Model file for the job. Use its own axes, mm. Face numbers are marked on the shaded views. A direction names the side the tool comes from. Round coordinates to 2 decimals unless told otherwise and drop trailing zeros. Write each loop counter-clockwise with the first axis right and the second up, starting at its lowest first coordinate (ties: lowest second). Pieces come first, ordered by that corner, then holes.
```python
from build123d import *

# Parameters (mm, degrees)
EXTRUDE_1_DEPTH     = 46.5
CUT_EXTRUDE_1_DEPTH = 87.088617134
CUT_EXTRUDE_2_DEPTH = 30
SKETCH_4_R          = 4
CUT_EXTRUDE_3_DEPTH = 100.36297097


with BuildPart() as part:
    # ｽｹｯﾁ1 → ﾎﾞｽ - 押し出し1 (new, symmetric)
    with BuildSketch(Plane.XY):
        Polygon((-65, 0), (65, 0), (35, 32), (-35, 32), align=None)
    extrude(amount=EXTRUDE_1_DEPTH, both=True)

    # ｽｹｯﾁ2 → ｶｯﾄ - 押し出し1 (cut, through all)
    with BuildSketch(Plane(origin=(0, 32, 0), x_dir=(1, 0, 0), z_dir=(0, 1, 0))):
        Polygon((-55, -46.5), (-35, -21.5), (35, -21.5), (55, -46.5), align=None)
        Polygon((-55, 46.5), (-35, 21.5), (35, 21.5), (55, 46.5), align=None)
    extrude(amount=-CUT_EXTRUDE_1_DEPTH, mode=Mode.SUBTRACT)

    # ｽｹｯﾁ3 → ｶｯﾄ - 押し出し2 (cut)
    with BuildSketch(Plane(origin=(0, 32, 0), x_dir=(1, 0, 0), z_dir=(0, 1, 0))):
        Polygon((-35.961249695, -19.5), (35.961249695, -19.5), (55.961249695, -44.5), (63, -44.5), (63, 44.5), (55.961249695, 44.5), (35.961249695, 19.5), (-35.961249695, 19.5), (-55.961249695, 44.5), (-63, 44.5), (-63, -44.5), (-55.961249695, -44.5), align=None)
    extrude(amount=-CUT_EXTRUDE_2_DEPTH, mode=Mode.SUBTRACT)

    # ｽｹｯﾁ4 → ｶｯﾄ - 押し出し3 (cut, through all)
    with BuildSketch(Plane.XY.offset(21.5)):
        with Locations((-17.5, 22)):
            Circle(SKETCH_4_R)
        with Locations((17.5, 22)):
            Circle(SKETCH_4_R)
    extrude(amount=-CUT_EXTRUDE_3_DEPTH, mode=Mode.SUBTRACT)


solid = part.part
```
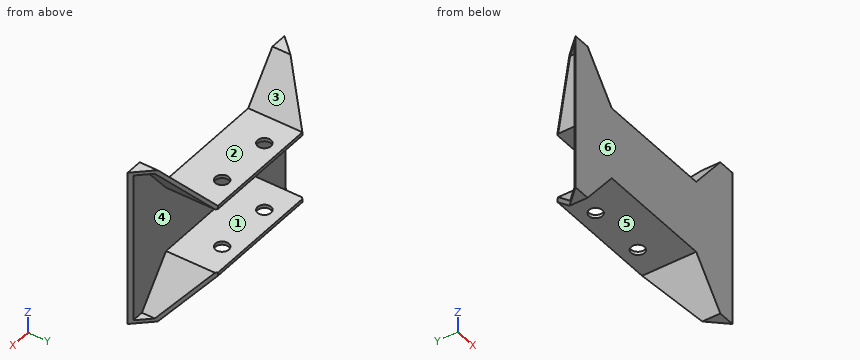
1) Cut at C-C on z = -24.5. List the corners of the cut face in (x, y).
2) Which spindle directions (+Z, -Z, +X, -X, +Y, -Y) get a long thin tool onto all of the face, cutting with end or side? Do the marked faces 3, 4, 5 and 6. Say none if no direction does.
3) Cut at B-B on y = 29. List the corners of the cut face in (x, z).
4) Flat gauge pins, fed straight in: pin 1 Ø5 at (x, y) = (17.5, 22) entering from -Z; pin 2 Ø13 at (x, y) = (-17.5, 22) entering from +Z; pin 3 Ø12 at (x, y) = (-14.5, 23) entering from -Z; pin 4 Ø1 at (y, z) = (12.5, 32) entering from +X. Where does each tip first touch, or does it go through?
5) Wall check: probe 1 along Z at (x, y) = (-10.5, 16.5); probe 2 along Y at (x, z) = (17, -20); probe 3 along Y at (x, z) = (-38, -17). Give the ranges that are in metal, low to high.
6) Cut at A-A on x = 17.5. List the corners of the cut face in (y, z).
7) Cut at D-D on y = 22. Give the number of separate pieces and of enclosed holes in the cut face, and give its area (3 significant figures).
8) Pull direction X, two halves, no side cores. Call the marked faces 1 and 2: released by +X, released by -X, zero draft, split by the parting line, or undercut.
Result sheet:
1. outline: (-65, 0) - (-37.4, 0) - (-37.4, 29.44) - (-39.96, 26.71) - (-39.96, 2) - (-63, 2) - (-63, 2.13) - close; (37.4, 0) - (65, 0) - (63, 2.13) - (63, 2) - (39.96, 2) - (39.96, 26.71) - (37.4, 29.44) - close
2. face 3: +Z, +Y, -Y
2. face 4: +Y
2. face 5: -Z, +Y, -Y
2. face 6: +Z, -Z, +X, -X, -Y
3. outline: (-37.81, -25.02) - (-35, -21.5) - (35, -21.5) - (37.81, -25.02) - (37.81, -21.81) - (35.96, -19.5) - (-35.96, -19.5) - (-37.81, -21.81) - close; (-37.81, 21.81) - (-35.96, 19.5) - (35.96, 19.5) - (37.81, 21.81) - (37.81, 25.02) - (35, 21.5) - (-35, 21.5) - (-37.81, 25.02) - close
4. pin 1: passes through
4. pin 2: stops at z = 21.5
4. pin 3: stops at z = -21.5
4. pin 4: stops at x = 46.36
5. probe 1: z = -21.5 to -19.5, 19.5 to 21.5
5. probe 2: y = 0 to 18.03, 25.97 to 32
5. probe 3: y = 0 to 2
6. outline: (0, -21.5) - (18, -21.5) - (18, -19.5) - (2, -19.5) - (2, 19.5) - (18, 19.5) - (18, 21.5) - (0, 21.5) - close; (26, -21.5) - (32, -21.5) - (32, -19.5) - (26, -19.5) - close; (26, 19.5) - (32, 19.5) - (32, 21.5) - (26, 21.5) - close
7. separate pieces: 6
7. enclosed holes: 0
7. area: 334 mm2
8. face 1: zero draft
8. face 2: undercut
